Autodesk Fusion 360 part; units mm, degrees
sketch "Sketch1" plane through (0, 0, 0) normal (0, 0, 1) x (1, 0, 0)
  line L0 (0, 0) -> (0, 57.5)
  line L1 (0, 57.5) -> (29.1254, 46.4677)
  line L2 (33, 40.8567) -> (33, -40.8567)
  line L3 (29.1254, -46.4677) -> (0, -57.5)
  line L4 (0, -57.5) -> (0, 0)
  arc A0 (29.1254, -46.4677) -> (33, -40.8567) centre (27, -40.8567) ccw
  arc A1 (33, 40.8567) -> (29.1254, 46.4677) centre (27, 40.8567) ccw
  point P0 (33, 45)
  point P1 (33, -45)
  dimension "d1" = 90
  dimension "d2" = 115
  dimension "d3" = 33
  dimension "d4" = 6
extrude "Extrude1" add sketch "Sketch1" along normal blind 3
sketch "Sketch2" plane through (0, 0, 3) normal (0, 0, 1) x (1, 0, 0)
  arc A0 (29.1254, -46.4677) -> (33, -40.8567) centre (27, -40.8567) ccw
  line L0 (33, -40.8567) -> (33, 40.8567)
  arc A1 (33, 40.8567) -> (29.1254, 46.4677) centre (27, 40.8567) ccw
  line L1 (29.1254, 46.4677) -> (0, 57.5)
  line L2 (0, 57.5) -> (0, -57.5)
  line L3 (0, -57.5) -> (29.1254, -46.4677)
  line L4 (23, -48.7879) -> (23, 48.7879) construction
  circle A2 centre (23, 0) radius 3.2
  circle A3 centre (23, 18) radius 1.5
  circle A4 centre (23, -18) radius 1.5
  dimension "d7" = 10
  dimension "d8" = 6.4
  dimension "d9" = 3
  dimension "d11" = 36
  dimension "d12" = 18
hole "Hole1" at (23, 0, 3) direction (0, 0, -1) diameter 6.4 end up to surface (3 mm away)
hole "Hole2" at (23, -18, 3) at (23, 18, 3) direction (0, 0, -1) diameter 3.5 depth 3 tip angle 118 counterbore diameter 5.5 counterbore depth 1.5
fillet "Fillet1" radius 1 10 edges at (14.5627, -51.9838, 3) (31.9372, -44.2661, 3) (33, 0, 3) (31.9372, 44.2661, 3) (14.5627, 51.9838, 3) (14.5627, 51.9838, 0) (31.9372, 44.2661, 0) (33, 0, 0) (31.9372, -44.2661, 0) (14.5627, -51.9838, 0)
equation "d8 = ( 25.6 / 4 ) * 1 mm"
Work out the finished part from the listing and answer in its coordinate system (mm). A direction names the side the tool comes from. Coordinates: 2 decimals unless noted, no trailing zeros. Loops run counter-clockwise (first coordinate to the right, second up) from the corner with the lowest first, then second, coordinate; pieces in that order, holes last. Notation, with made-up numbers: M 12.25,-9.75 L 26.25,-9.75 A36 cw 26.25,29.25 Z; hole C 60,-21 d5. An arc over 180 degrees is marked long. Answer in a Markdown table with one row per item. Add a question column.
1. Flat-ended cylindrical pins translate along their axes: P1, Ø7, axis at x = 23, y = 18, coming from the -Z side; P2, Ø1.6, axis at x = 21.5, y = -18, coming from the +Z side; P3, Ø1.5, axis at x = 15.5, z = 1.5, coming from the -Y side; P4, Ø3, axis at x = 23, y = -18, coming from the +Z side. Find the tip coordinate at first contact, or state that the pin passes through.
2. Consider L1, parallel to Y at x = 23, z = 2.6; L2, parallel to X at y = 18, z = 0.8; L3, parallel to Y at x = 23, z = 2.35. Determine where each line is inside the solid, lowest interval first.
3. Find section A-A, the plane y = -18. Write down the section's boundary in (x, z).
4. A tool of negligible diameter and unlimited length cuts with its end or side. For faces 1 (the flat face through (16, 1, 3)), 2 (the cylindrical face through (22.879, 20.747, 2.24)), from which of +Z, -Z, +X, -X, +Y, -Y can it reach the whole face along a straight path? Write none if from no direction.
5. Find section B-B, the plane y = 0. Write down the section's boundary in (x, z).
6. Find section C-C, the plane x = 23. State how many separate pieces and enclosed holes the cut face has, then the cut area to 3 significant figures.
Reported:
| question | item | result |
|---|---|---|
| 1 | P1 | stops at z = 0 |
| 1 | P2 | stops at z = 1.5 |
| 1 | P3 | stops at y = -51.91 |
| 1 | P4 | passes through |
| 2 | L1 | y = -48.57 to -20.75, -15.25 to -3.2, 3.2 to 15.25, 20.75 to 48.57 |
| 2 | L2 | x = 0 to 21.25, 24.75 to 32.98 |
| 2 | L3 | y = -48.72 to -20.75, -15.25 to -3.2, 3.2 to 15.25, 20.75 to 48.72 |
| 3 | outline | M 0,0 L 21.25,0 L 21.25,1.5 L 20.25,1.5 L 20.25,3 L 0,3 Z; M 24.75,0 L 32,0 A1 ccw 33,1 L 33,2 A1 ccw 32,3 L 25.75,3 L 25.75,1.5 L 24.75,1.5 Z |
| 4 | face 1 | +Z, +X, -X, +Y, -Y |
| 4 | face 2 | +Z |
| 5 | outline | M 0,0 L 19.8,0 L 19.8,3 L 0,3 Z; M 26.2,0 L 32,0 A1 ccw 33,1 L 33,2 A1 ccw 32,3 L 26.2,3 Z |
| 6 | separate pieces | 4 |
| 6 | enclosed holes | 0 |
| 6 | area | 246 mm^2 |
